Could you check a few things on this model? Use its own coordinates, in mm. Face numbers are marked on the shaded views. A direction names the side the tool comes from. Round coordinates to 2 decimals unless told otherwise and drop trailing zeros. Write each loop counter-clockwise with the first axis right and the second up, starting at its lowest first coordinate (ties: lowest second). Pieces come first, ordered by that corner, then holes. Notation, with made-up numbers: (69, 26) -> (88, 26) arc R17 ccw to (88, 40) -> close; hole circle Ø9 at (54, -36). An arc over 180 degrees is marked (long way). Answer in a Markdown table with one row per item. Add a question column.
```python
from build123d import *

# Parameters (mm, degrees)
BOSS_EXTRUDE1_DEPTH = 15
CUT_EXTRUDE1_DEPTH  = 16
SKETCH3_W           = 50
SKETCH3_H           = 45
BOSS_EXTRUDE3_DEPTH = 15
SKETCH4_W           = 12.5
SKETCH4_H           = 6.523729489
CUT_EXTRUDE2_DEPTH  = 4
FILLET1_R           = 2
SKETCH5_W           = 50
SKETCH5_H           = 25
SKETCH5_R           = 7.5
BOSS_EXTRUDE4_DEPTH = 15
SKETCH6_R           = 2
CUT_EXTRUDE3_DEPTH  = 16
BOSS_EXTRUDE5_DEPTH = 5
SKETCH8_W           = 50
SKETCH8_H           = 93.984880812
BOSS_EXTRUDE6_DEPTH = 5
SKETCH9_R           = 2
SKETCH9_R_2         = 7.5
CUT_EXTRUDE4_DEPTH  = 21
SKETCH10_R          = 2
CUT_EXTRUDE5_DEPTH  = 21


with BuildPart() as part:
    # Sketch1 → Boss-Extrude1 (new body)
    with BuildSketch(Plane.XY):
        with BuildLine():
            Line((-7, 19), (7, 19))
            ThreePointArc((7, 19), (14.071067812, 16.071067812), (17, 9))
            Line((17, 9), (17, -5))
            ThreePointArc((17, -5), (14.071067812, -12.071067812), (7, -15))
            Line((7, -15), (-7, -15))
            ThreePointArc((-7, -15), (-14.071067812, -12.071067812), (-17, -5))
            Line((-17, -5), (-17, 9))
            ThreePointArc((-17, 9), (-14.071067812, 16.071067812), (-7, 19))
        make_face()
    extrude(amount=BOSS_EXTRUDE1_DEPTH)

    # Sketch2 → Cut-Extrude1 (cut, through all)
    with BuildSketch(Plane(origin=(0, 0, 0), x_dir=(-1, 0, 0), z_dir=(0, 0, -1))):
        with BuildLine():
            Line((14, 0.39), (14, 8.212908396))
            ThreePointArc((14, 8.212908396), (11.719213675, 13.719213675), (6.212908396, 16))
            Line((6.212908396, 16), (-6.212908396, 16))
            ThreePointArc((-6.212908396, 16), (-11.719213675, 13.719213675), (-14, 8.212908396))
            Line((-14, 8.212908396), (-14, 0.39))
            Line((-14, 0.39), (-14, -2.4))
            ThreePointArc((-14, -2.4), (-12.535533906, -5.935533906), (-9, -7.4))
            Line((-9, -7.4), (-8.25, -7.4))
            ThreePointArc((-8.25, -7.4), (-6.835786438, -7.985786438), (-6.25, -9.4))
            Line((-6.25, -9.4), (-6.25, -17.62539529))
            Line((-6.25, -17.62539529), (6.25, -17.62539529))
            Line((6.25, -17.62539529), (6.25, -9.4))
            ThreePointArc((6.25, -9.4), (6.835786438, -7.985786438), (8.25, -7.4))
            Line((8.25, -7.4), (9, -7.4))
            ThreePointArc((9, -7.4), (12.535533906, -5.935533906), (14, -2.4))
            Line((14, -2.4), (14, 0.39))
        make_face()
    extrude(amount=-CUT_EXTRUDE1_DEPTH, mode=Mode.SUBTRACT)

    # Sketch3 → Boss-Extrude3 (add)
    with BuildSketch(Plane(origin=(0, 0, 0), x_dir=(-1, 0, 0), z_dir=(0, 0, -1))):
        with Locations((0, -0.507559594)):
            Rectangle(SKETCH3_W, SKETCH3_H)
        with BuildLine():
            Line((-6.25, -9.4), (-6.25, -15))
            Line((-6.25, -15), (-6.25, -17.5))
            ThreePointArc((-6.25, -17.5), (-5.664213562, -18.914213562), (-4.25, -19.5))
            Line((-4.25, -19.5), (4.25, -19.5))
            ThreePointArc((4.25, -19.5), (5.664213562, -18.914213562), (6.25, -17.5))
            Line((6.25, -17.5), (6.25, -15))
            Line((6.25, -15), (6.25, -9.4))
            ThreePointArc((6.25, -9.4), (6.835786438, -7.985786438), (8.25, -7.4))
            Line((8.25, -7.4), (9, -7.4))
            ThreePointArc((9, -7.4), (12.535533906, -5.935533906), (14, -2.4))
            Line((14, -2.4), (14, 8.212908396))
            ThreePointArc((14, 8.212908396), (11.719213675, 13.719213675), (6.212908396, 16))
            Line((6.212908396, 16), (-6.212908396, 16))
            ThreePointArc((-6.212908396, 16), (-11.719213675, 13.719213675), (-14, 8.212908396))
            Line((-14, 8.212908396), (-14, -2.4))
            ThreePointArc((-14, -2.4), (-12.535533906, -5.935533906), (-9, -7.4))
            Line((-9, -7.4), (-8.25, -7.4))
            ThreePointArc((-8.25, -7.4), (-6.835786438, -7.985786438), (-6.25, -9.4))
        make_face(mode=Mode.SUBTRACT)
    extrude(amount=-BOSS_EXTRUDE3_DEPTH)

    # Sketch4 → Cut-Extrude2 (cut)
    with BuildSketch(Plane(origin=(0, 0, 0), x_dir=(-1, 0, 0), z_dir=(0, 0, -1))):
        with Locations((0, -19.74569485)):
            Rectangle(SKETCH4_W, SKETCH4_H)
    extrude(amount=-CUT_EXTRUDE2_DEPTH, mode=Mode.SUBTRACT)

    # Fillet1
    fillet1_edges = [part.edges().sort_by_distance(p)[0] for p in [
        (6.25, -23.007559594, 2),
        (-6.25, -23.007559594, 2),
    ]]
    fillet(fillet1_edges, radius=FILLET1_R)

    # Sketch5 → Boss-Extrude4 (add)
    with BuildSketch(Plane.XY.offset(15)):
        with Locations((0, 34.492440406)):
            Rectangle(SKETCH5_W, SKETCH5_H)
        with Locations((0, 34.492440406)):
            Circle(SKETCH5_R, mode=Mode.SUBTRACT)
    boss_extrude4 = extrude(amount=-BOSS_EXTRUDE4_DEPTH)

    # Mirror1: Boss-Extrude4 across plane
    add(boss_extrude4.mirror(Plane.ZX))

    # Sketch6 → Cut-Extrude3 (cut, through all)
    with BuildSketch(Plane.XY.offset(15)):
        with Locations((-20, 41.992440406)):
            Circle(SKETCH6_R)
        with Locations((20, 41.992440406)):
            Circle(SKETCH6_R)
        with Locations((20, -41.992440406)):
            Circle(SKETCH6_R)
        with Locations((-20, -41.992440406)):
            Circle(SKETCH6_R)
        with Locations((20, 0)):
            Circle(SKETCH6_R)
        with Locations((-20, 0)):
            Circle(SKETCH6_R)
    extrude(amount=-CUT_EXTRUDE3_DEPTH, mode=Mode.SUBTRACT)

    # Sketch7 → Boss-Extrude5 (add)
    with BuildSketch(Plane.XY.offset(15)):
        with BuildLine():
            Line((-4.25, -19.5), (4.25, -19.5))
            ThreePointArc((4.25, -19.5), (5.664213562, -18.914213562), (6.25, -17.5))
            Line((6.25, -17.5), (6.25, -9.4))
            ThreePointArc((6.25, -9.4), (6.835786438, -7.985786438), (8.25, -7.4))
            Line((8.25, -7.4), (9, -7.4))
            ThreePointArc((9, -7.4), (12.535533906, -5.935533906), (14, -2.4))
            Line((14, -2.4), (14, 8.212908396))
            ThreePointArc((14, 8.212908396), (11.719213675, 13.719213675), (6.212908396, 16))
            Line((6.212908396, 16), (-6.212908396, 16))
            ThreePointArc((-6.212908396, 16), (-11.719213675, 13.719213675), (-14, 8.212908396))
            Line((-14, 8.212908396), (-14, -2.4))
            ThreePointArc((-14, -2.4), (-12.535533906, -5.935533906), (-9, -7.4))
            Line((-9, -7.4), (-8.25, -7.4))
            ThreePointArc((-8.25, -7.4), (-6.835786438, -7.985786438), (-6.25, -9.4))
            Line((-6.25, -9.4), (-6.25, -17.5))
            ThreePointArc((-6.25, -17.5), (-5.664213562, -18.914213562), (-4.25, -19.5))
        make_face()
    extrude(amount=-BOSS_EXTRUDE5_DEPTH)

    # Sketch8 → Boss-Extrude6 (add)
    with BuildSketch(Plane.XY.offset(15)):
        Rectangle(SKETCH8_W, SKETCH8_H)
    extrude(amount=BOSS_EXTRUDE6_DEPTH)

    # Sketch9 → Cut-Extrude4 (cut, through all)
    with BuildSketch(Plane(origin=(0, 0, 0), x_dir=(-1, 0, 0), z_dir=(0, 0, -1))):
        with Locations((20, -41.992440406)):
            Circle(SKETCH9_R)
        with Locations((0, -34.492440406)):
            Circle(SKETCH9_R_2)
        with Locations((-20, -41.992440406)):
            Circle(SKETCH9_R)
        with Locations((20, 0)):
            Circle(SKETCH9_R)
        with Locations((-20, 0)):
            Circle(SKETCH9_R)
        with Locations((-20, 41.992440406)):
            Circle(SKETCH9_R)
        with Locations((0, 34.492440406)):
            Circle(SKETCH9_R_2)
        with Locations((20, 41.992440406)):
            Circle(SKETCH9_R)
    extrude(amount=-CUT_EXTRUDE4_DEPTH, mode=Mode.SUBTRACT)

    # Sketch10 → Cut-Extrude5 (cut, through all)
    with BuildSketch(Plane.XY.offset(20)):
        with Locations((-20, 24.492440406)):
            Circle(SKETCH10_R)
        with Locations((20, 24.492440406)):
            Circle(SKETCH10_R)
        with Locations((20, -24.492440406)):
            Circle(SKETCH10_R)
        with Locations((-20, -24.492440406)):
            Circle(SKETCH10_R)
    extrude(amount=-CUT_EXTRUDE5_DEPTH, mode=Mode.SUBTRACT)


solid = part.part
```
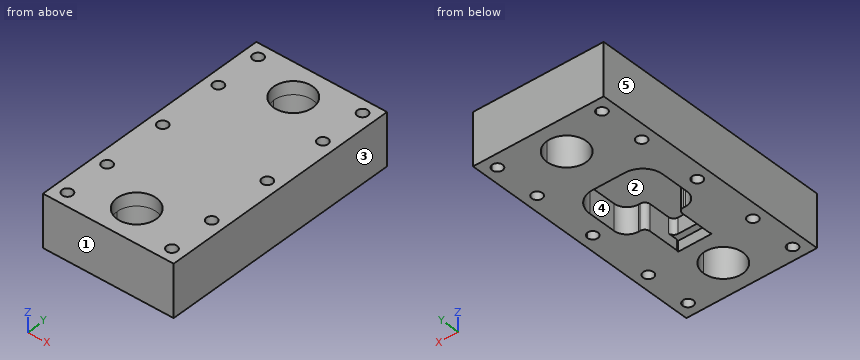
(1) Suppose I cut it at A-A, the plane x = -20. Please give me the cut outline in (y, z).
(2) For P1, Ø5, axis at x = 20, y = -24.49, coming from the -Z side; P2, Ø13.5, axis at x = 0, y = -34.49, coming from the -Z side (3 decimals); P3, Ø3.5, axis at x = 0, y = -19.5, coming from the -Z side, each with a flat end and sliding along its axis, tell me the tip position at first contact or that it passes through.
(3) Suppose I cut it at D-D, the plane z = 8. State how many separate pieces and enclosed holes the cut face has, then the cut area to 3 significant figures.
(4) Suppose I cut it at B-B, the plane x = 0. Please give me the cut outline in (y, z).
(5) On a 3-axis mill with a long thin cutter (end or side, diameter ignored), from which of +Z, -Z, +X, -X, +Y, -Y can I reach the whole of each face in a straight line? I mean the marked faces 1 and 2. Say none if no direction works.
(6) Suppose I cut it at C-C, the plane y = -33. Please give me the cut outline in (x, z).
(7) If we mould it in two halves opening along X, with no side actions, what happens to the marked faces 3, 4 and 5? For each: pulls with the +X half, pulls with the -X half, needs draft (parallel to the pull), parting line crosses it, or undercut.
(8) I need wall thicknesses on L1, parallel to Y at x = 20, z = 6.5; L2, parallel to X at y = 0, z = 16.8; L3, parallel to Y at x = 0, z = 16.4. Which ranges of each line are inside material? Lowest first, please.
Response:
| question | item | result |
|---|---|---|
| 1 | outline | (-46.99, 0) -> (-43.99, 0) -> (-43.99, 20) -> (-46.99, 20) -> close; (-39.99, 0) -> (-26.49, 0) -> (-26.49, 20) -> (-39.99, 20) -> close; (-22.49, 0) -> (-2, 0) -> (-2, 20) -> (-22.49, 20) -> close; (2, 0) -> (22.49, 0) -> (22.49, 20) -> (2, 20) -> close; (26.49, 0) -> (39.99, 0) -> (39.99, 20) -> (26.49, 20) -> close; (43.99, 0) -> (46.99, 0) -> (46.99, 20) -> (43.99, 20) -> close |
| 2 | P1 | z = 0 |
| 2 | P2 | through |
| 2 | P3 | z = 4 |
| 3 | separate pieces | 1 |
| 3 | enclosed holes | 13 |
| 3 | area | 3,450 mm² |
| 4 | outline | (-46.99, 0) -> (-41.99, 0) -> (-41.99, 20) -> (-46.99, 20) -> close; (-26.99, 0) -> (-21.99, 0) -> (-21.99, 4) -> (-19.5, 4) -> (-19.5, 10) -> (16, 10) -> (16, 0) -> (26.99, 0) -> (26.99, 20) -> (-26.99, 20) -> close; (41.99, 0) -> (46.99, 0) -> (46.99, 20) -> (41.99, 20) -> close |
| 5 | face 1 | +Z, -Z, +X, -X, -Y |
| 5 | face 2 | -Z |
| 6 | outline | (-25, 0) -> (-7.35, 0) -> (-7.35, 20) -> (-25, 20) -> close; (7.35, 0) -> (25, 0) -> (25, 20) -> (7.35, 20) -> close |
| 7 | face 3 | pulls with the +X half |
| 7 | face 4 | undercut |
| 7 | face 5 | pulls with the -X half |
| 8 | L1 | -46.99 to -43.99, -39.99 to -26.49, -22.49 to -2, 2 to 22.49, 26.49 to 39.99, 43.99 to 46.99 |
| 8 | L2 | -25 to -22, -18 to 18, 22 to 25 |
| 8 | L3 | -46.99 to -41.99, -26.99 to 26.99, 41.99 to 46.99 |
